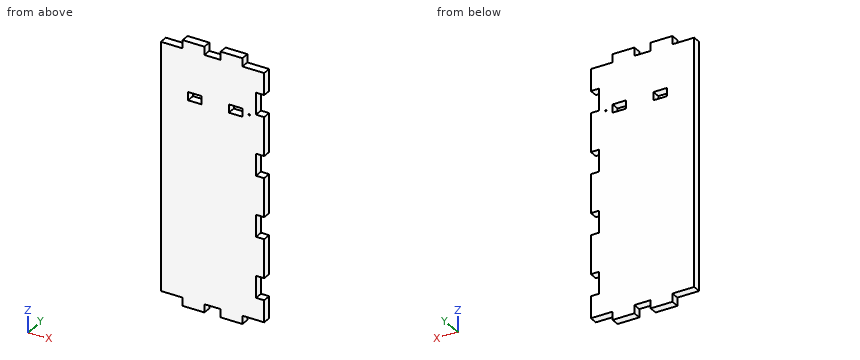
```python
from build123d import *

# Parameters (mm, degrees)
SKETCH1_W           = 60
SKETCH1_H           = 193
SKETCH1_W_2         = 10
BOSS_EXTRUDE1_DEPTH = 6
SKETCH4_W           = 6
SKETCH4_H           = 193
BOSS_EXTRUDE2_DEPTH = 6
SKETCH5_W           = 6
SKETCH5_H           = 16
SKETCH5_W_2         = 16
SKETCH5_H_2         = 6
SKETCH5_W_3         = 12
CUT_EXTRUDE1_DEPTH  = 7
SKETCH6_R           = 0.5
SKETCH6_W           = 10
SKETCH6_H           = 6
CUT_EXTRUDE2_DEPTH  = 7


with BuildPart() as part:
    # Sketch1 → Boss-Extrude1 (new body)
    with BuildSketch(Plane(origin=(0, 0, 0), x_dir=(1, 0, 0), z_dir=(0, 1, 0))):
        with Locations((5, 0)):
            Rectangle(SKETCH1_W, SKETCH1_H)
        with Locations((-30, 0)):
            Rectangle(SKETCH1_W_2, SKETCH1_H)
    extrude(amount=BOSS_EXTRUDE1_DEPTH)

    # Sketch4 → Boss-Extrude2 (add)
    with BuildSketch(Plane(origin=(0, 6, 0), x_dir=(1, 0, 0), z_dir=(0, 1, 0))):
        with Locations((38, 0)):
            Rectangle(SKETCH4_W, SKETCH4_H)
    extrude(amount=-BOSS_EXTRUDE2_DEPTH)

    # Sketch5 → Cut-Extrude1 (cut, through all)
    with BuildSketch(Plane(origin=(0, 6, 0), x_dir=(1, 0, 0), z_dir=(0, 1, 0))):
        with Locations((38, -66.5)):
            Rectangle(SKETCH5_W, SKETCH5_H)
        Polygon((35, -30.166666667), (41, -30.166666667), (41, -14.166666667), (38, -14.166666667), (35, -14.166666667), align=None)
        with Locations((33, -93.5)):
            Rectangle(SKETCH5_W_2, SKETCH5_H_2)
        with Locations((-27, -93.5)):
            Rectangle(SKETCH5_W_2, SKETCH5_H_2)
        with Locations((3, -93.5)):
            Rectangle(SKETCH5_W_3, SKETCH5_H_2)
    cut_extrude1 = extrude(amount=-CUT_EXTRUDE1_DEPTH, mode=Mode.SUBTRACT)

    # Mirror1: Cut-Extrude1 across plane
    add(cut_extrude1.mirror(Plane.XY), mode=Mode.SUBTRACT)

    # Sketch6 → Cut-Extrude2 (cut, through all)
    with BuildSketch(Plane(origin=(0, 6, 0), x_dir=(1, 0, 0), z_dir=(0, 1, 0))):
        with Locations((30, -57)):
            Circle(SKETCH6_R)
        with Locations((20, -57)):
            Rectangle(SKETCH6_W, SKETCH6_H)
        with Locations((-10, -57)):
            Rectangle(SKETCH6_W, SKETCH6_H)
    extrude(amount=-CUT_EXTRUDE2_DEPTH, mode=Mode.SUBTRACT)


solid = part.part
```
Read the model definition and answer for the solid it produces. Units are mm, in the model's axes. Round coordinates to 2 decimals unless told otherwise and drop trailing zeros. Write each loop counter-clockwise with the first axis right and the second up, starting at its lowest first coordinate (ties: lowest second). Pieces come first, ordered by that corner, then holes. Notation, with made-up numbers: (28, -13) - (48, -13) arc R31 cw to (48, 19) - close; hole circle Ø7 at (-33.5, 24). An arc over 180 degrees is marked (long way). One line per item, written item: value.
Q1. Find section D-D (x = -26). Determine the outline of the cut face in (y, z).
The answers:
outline: (0, -90.5) - (6, -90.5) - (6, 90.5) - (0, 90.5) - close
Q2. Straight lines are drawn through the part: line 1 (X direction, y = 1.35, z = 57); line 2 (Z direction, x = 24, y = 2.4); line 3 (Z direction, x = 30, y = 4.15). For each, find the intervals that lie inside material, in ascending order. Write a range as from..to.
The answers:
line 1: x = -35..-15, -5..15, 25..29.5, 30.5..41
line 2: z = -96.5..54, 60..96.5
line 3: z = -90.5..56.5, 57.5..90.5
Q3. Find section C-C (y = 3.65). Count the separate pieces of the cut face and the enclosed holes in it, and give its area (3 significant figures).
The answers:
separate pieces: 1
enclosed holes: 3
area: 13,600 mm2
Q4. Find section B-B (z = -65). Determine the outline of the cut face in (x, y), and give its area (3 significant figures).
The answers:
outline: (-35, 0) - (35, 0) - (35, 6) - (-35, 6) - close
area: 420 mm2
Q5. Each of these flat-tipped pins is pushed along its axis until it touches: P1, Ø3, axis at y = 4, z = -93.5, coming from the +X side; P2, Ø1.8, axis at y = 3, z = -92.5, coming from the -X side; P3, Ø1.8, axis at x = 29.5, y = 2.5, coming from the +Z side. Where does it stop, or does it pass through?
The answers:
P1: stops at x = 25
P2: stops at x = -19
P3: stops at z = 90.5
Q6. Find section A-A (x = -10). Determine the outline of the cut face in (y, z), and give its area (3 significant figures).
The answers:
outline: (0, -96.5) - (6, -96.5) - (6, 54) - (0, 54) - close; (0, 60) - (6, 60) - (6, 96.5) - (0, 96.5) - close
area: 1,120 mm2
